The model under review builds one solid part; all positions refer to its coordinate system, in mm. A direction names the side the tool comes from. Round coordinates to 2 decimals unless told otherwise and drop trailing zeros. Order: outer loops, then holes, each group sorted by start corner. A loop starts at its lowest first (then second) coordinate and runs counter-clockwise, first axis right, second up. Notation, with made-up numbers: M 47,31.25 L 68,31.25 A16 cw 68,48.25 Z; hole C -32.75,-6 d6. An arc over 180 degrees is marked long. One line per item, written item: value. Start each with the question number.
from build123d import *

# Parameters (mm, degrees)
BOSS_EXTRUDE1_DEPTH = 2.032
SKETCH2_R           = 1.016
SKETCH2_R_2         = 0.635
CUT_EXTRUDE1_DEPTH  = 3.032
SKETCH3_W           = 6.145312949
SKETCH3_H           = 3.136404534
BOSS_EXTRUDE2_DEPTH = 1.27


with BuildPart() as part:
    # Sketch1 → Boss-Extrude1 (new body)
    with BuildSketch(Plane(origin=(0, 0, 0), x_dir=(1, 0, 0), z_dir=(0, 1, 0))):
        with BuildLine():
            Line((0, 2.54), (0, 16.51))
            ThreePointArc((0, 16.51), (0.743948776, 18.306051224), (2.54, 19.05))
            Line((2.54, 19.05), (16.51, 19.05))
            ThreePointArc((16.51, 19.05), (18.306051224, 18.306051224), (19.05, 16.51))
            Line((19.05, 16.51), (19.05, 2.54))
            ThreePointArc((19.05, 2.54), (18.306051224, 0.743948776), (16.51, 0))
            Line((16.51, 0), (2.54, 0))
            ThreePointArc((2.54, 0), (0.743948776, 0.743948776), (0, 2.54))
        make_face()
    extrude(amount=BOSS_EXTRUDE1_DEPTH)

    # Sketch2 → Cut-Extrude1 (cut, through all)
    with BuildSketch(Plane(origin=(0, 2.032, 0), x_dir=(1, 0, 0), z_dir=(0, 1, 0))):
        with Locations((2.54, 16.51)):
            Circle(SKETCH2_R)
        with Locations((16.51, 16.51)):
            Circle(SKETCH2_R)
        with Locations((2.54, 2.54)):
            Circle(SKETCH2_R_2)
        with Locations((4.868333333, 2.54)):
            Circle(SKETCH2_R_2)
        with Locations((7.196666667, 2.54)):
            Circle(SKETCH2_R_2)
        with Locations((9.525, 2.54)):
            Circle(SKETCH2_R_2)
        with Locations((11.853333333, 2.54)):
            Circle(SKETCH2_R_2)
        with Locations((14.181666667, 2.54)):
            Circle(SKETCH2_R_2)
        with Locations((16.51, 2.54)):
            Circle(SKETCH2_R_2)
    extrude(amount=-CUT_EXTRUDE1_DEPTH, mode=Mode.SUBTRACT)

    # Sketch3 → Boss-Extrude2 (add)
    with BuildSketch(Plane(origin=(0, 2.032, 0), x_dir=(1, 0, 0), z_dir=(0, 1, 0))):
        with Locations((9.384754269, 10.047734089)):
            Rectangle(SKETCH3_W, SKETCH3_H)
    extrude(amount=BOSS_EXTRUDE2_DEPTH)


solid = part.part
Item 1: Clearance check with a flat-ended pin moving along its axis: P1, Ø2, axis at x = 9.525, z = -2.54, coming from the +Y side. State where the tip first meets the part, or that it passes through.
Item 2: The part is to be moulded in two halves that separate along Z. For faces 6 (the cylindrical face through (7.783, 1.03, -2.297)), 7 (the flat face through (10, 1, 0)), 8 (the cylindrical face through (17.1, 1, -2.3)), 9 (the flat face through (0, 1, -9)), say which applies: pulls with the +Z half, pulls with the -Z half, needs draft (parallel to the pull), parting line crosses it, or undercut.
Item 3: Consider section D-D, the plane y = 2.4. Give the boundary of the cut face in (x, z).
Item 4: Wall thickness on L1, parallel to Z at x = 16.51, y = 1.15 (3 decimals); L2, parallel to X at y = 1.3, z = -16.51; L3, parallel to Y at x = 14.5, z = -6: over which ranges is each line inside the solid? List them lowest first.
Item 5: Consider section A-A, the plane y = 0.35. Count the separate pieces of the cut face and the enclosed holes in it, then the cut area to 3 significant figures.
Item 6: Consider section C-C, the plane z = -13. Give the boundary of the cut face in (x, y), then the cut area to 3 significant figures.
Item 7: Machinability: for faces 1 (the flat face through (9, 3, -8.48)), 2 (the flat face through (12.457, 3, -10)), 3 (the flat face through (6.312, 3, -10)), 4 (the cylindrical face through (18.326, 1.002, -0.764)), 5 (the cylindrical face through (14.475, 1.03, -1.977)), which of the approach directions +Z, -Z, +X, -X, +Y, -Y give a long, thin tool a straight path to every point of the face, cutting with its end or side? Answer none if there is none.
Computed:
1. P1: stops at y = 2.03
2. face 6: undercut
2. face 7: pulls with the +Z half
2. face 8: undercut
2. face 9: needs draft
3. outline: M 6.31,-11.62 L 12.46,-11.62 L 12.46,-8.48 L 6.31,-8.48 Z
4. L1: z = -19.05 to -17.526, -15.494 to -3.175, -1.905 to 0
4. L2: x = 0 to 1.52, 3.56 to 15.49, 17.53 to 19.05
4. L3: y = 0 to 2.03
5. separate pieces: 1
5. enclosed holes: 9
5. area: 342 mm^2
6. outline: M 0,0 L 19.05,0 L 19.05,2.03 L 0,2.03 Z
6. area: 38.7 mm^2
7. face 1: +Z, +X, -X, +Y
7. face 2: +Z, -Z, +X, +Y
7. face 3: +Z, -Z, -X, +Y
7. face 4: +Z, +X, +Y, -Y
7. face 5: +Y, -Y
